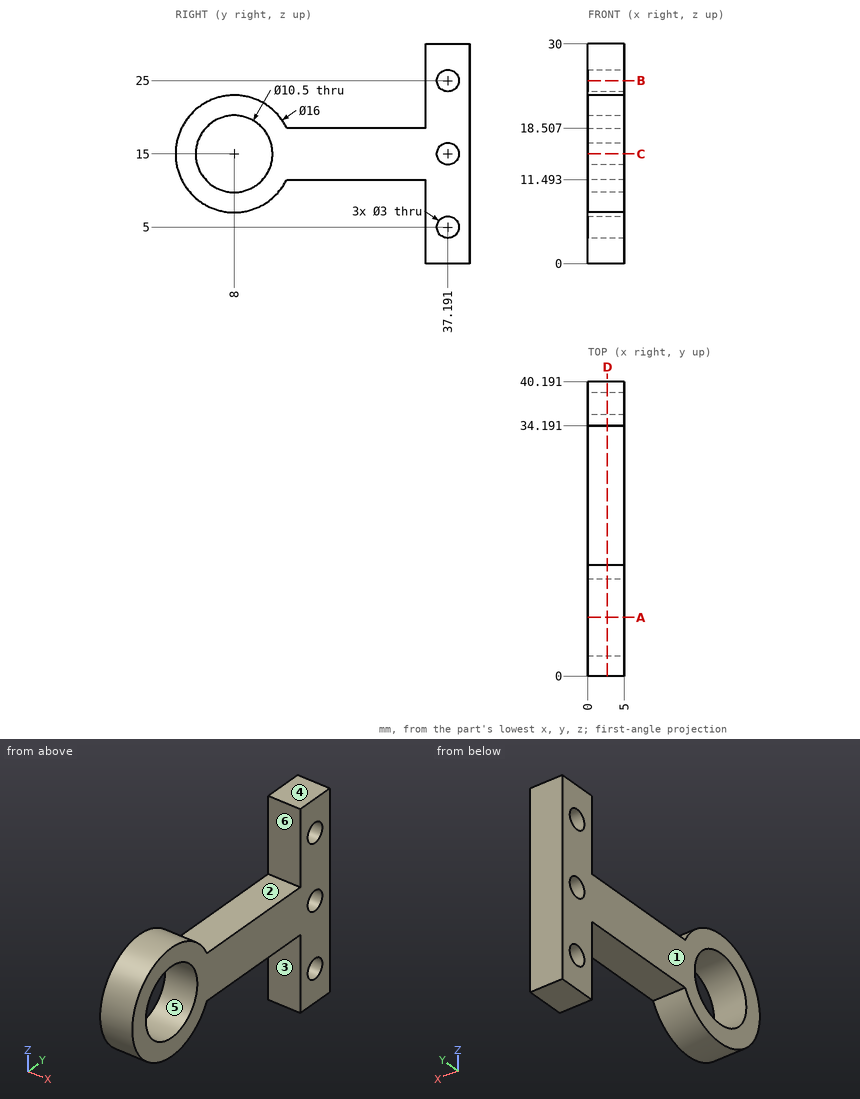
The figure shows three views and two pictorial views of one solid part (mm, origin at its lowest corner). Answer the questions. A direction names the side the tool comes from. Round coordinates to 2 decimals unless told otherwise and drop trailing zeros. Loops run counter-clockwise (first coordinate to the right, second up) from the corner with the lowest first, then second, coordinate; pieces in that order, holes last. Notation, with made-up numbers: M 76.25,33 L 120.25,33 A31 ccw 120.25,57 Z; hole C -37,7 d1. An arc over 180 degrees is marked long. Return JSON: item names as keys, results as strings.
Q1. Which of the six approach directions +Z, -Z, +X, -X, +Y, -Y give full straight-line access (tool end or side, diameter ignored) to the marked faces 1, 2 and 3?
Results list:
{"face 1": "+Z, -Z, -X, +Y, -Y", "face 2": "+Z, +X, -X", "face 3": "-Z, +X, -X"}
Q2. Find the intervals of material crossed by line 1 along Y through (x, z) = (2.9, 15); line 2 along Y through (x, z) = (1.85, 25); line 3 along Y through (x, z) = (3.5, 16) (1 decimal), in increasing order. Write a range as from..to.
Results list:
{"line 1": "y = 0..2.75, 13.25..35.69, 38.69..40.19", "line 2": "y = 34.19..35.69, 38.69..40.19", "line 3": "y = 0.1..2.8, 13.2..36.1, 38.3..40.2"}
Q3. The mould has two halves that part along Z. Classify the marked faces 4, 5 and 6: released by +Z, released by -Z, zero draft, split by the parting line, or undercut.
Results list:
{"face 4": "released by +Z", "face 5": "undercut", "face 6": "zero draft"}
Q4. Each of these flat-tipped pins is pushed along its axis until it touches: pin 1 Ø1 at (y, z) = (13.5, 20) entering from -X; pin 2 Ø2.5 at (x, z) = (1.5, 5) entering from -Y; pin 3 Ø2.5 at (x, y) = (2.5, 25) entering from +Z; pin 4 Ø3 at (x, z) = (2.5, 12.5) entering from -Y. Where does it stop, or does it pass through?
Results list:
{"pin 1": "stops at x = 0", "pin 2": "stops at y = 34.19", "pin 3": "stops at z = 18.51", "pin 4": "stops at y = 0.06"}
Q5. Find section B-B, the plane z = 25. Determine the outline of the cut face in (x, y).
Results list:
{"outline": "M 0,34.19 L 5,34.19 L 5,35.69 L 0,35.69 Z; M 0,38.69 L 5,38.69 L 5,40.19 L 0,40.19 Z"}
Q6. Find section C-C, the plane z = 15. Determine the outline of the cut face in (x, y).
Results list:
{"outline": "M 0,0 L 5,0 L 5,2.75 L 0,2.75 Z; M 0,13.25 L 5,13.25 L 5,35.69 L 0,35.69 Z; M 0,38.69 L 5,38.69 L 5,40.19 L 0,40.19 Z"}
Q7. Find section D-D, the plane x = 2.65. Determine the outline of the cut face in (y, z).
Results list:
{"outline": "M 15.19,11.49 L 34.19,11.49 L 34.19,0 L 40.19,0 L 40.19,30 L 34.19,30 L 34.19,18.51 L 15.19,18.51 A8 ccw long Z; hole C 8,15 d10.5; hole C 37.19,5 d3; hole C 37.19,15 d3; hole C 37.19,25 d3"}
Q8. Find section A-A, the plane y = 8. Determine the outline of the cut face in (x, z), plus the area to 3 significant figures.
Results list:
{"outline": "M 0,7 L 5,7 L 5,9.75 L 0,9.75 Z; M 0,20.25 L 5,20.25 L 5,23 L 0,23 Z", "area": "27.5 mm2"}
